from build123d import *

# Parameters (mm, degrees)
F0_W     = 30
F0_H     = 20
F1_DEPTH = 40
F2_R     = 4.672603
F3_DEPTH = 25
F4_R     = 2


with BuildPart() as f1:
    # F0 (on Top) → F1 (new body)
    with BuildSketch(Plane.XY):
        with Locations((15, 10)):
            Rectangle(F0_W, F0_H)
    extrude(amount=F1_DEPTH)

    # F2 (on face) → F3 (join)
    with BuildSketch(Plane.XY.offset(40)):
        with Locations((15, 10)):
            Circle(F2_R)
    extrude(amount=F3_DEPTH)

    # F4
    f4_edges = [f1.edges().sort_by_distance(p)[0] for p in [
        (10.327397, 10, 65),
        (30, 10, 40),
        (15, 0, 40),
        (0, 10, 40),
        (15, 20, 40),
        (30, 20, 20),
        (30, 0, 20),
        (0, 0, 20),
        (0, 20, 20),
    ]]
    fillet(f4_edges, radius=F4_R)


solid = f1.part
Verification items for the finished model (mm, model axes). A direction names the side the tool comes from. Coordinates: 2 decimals unless noted, no trailing zeros. Order: outer loops, then holes, each group sorted by start corner. A loop starts at its lowest first (then second) coordinate and runs counter-clockwise, first axis right, second up.
1. Sectioned sample at D-D, the plane y = 3.5. Record the cut outline in (x, z).
Results found:
outline: (0, 0) - (30, 0) - (30, 38) arc R2 ccw to (28, 40) - (2, 40) arc R2 ccw to (0, 38) - close
2. Set-up check for faces 1 (the face through (15, 0, 19)), 2 (the face through (14.392, 14.633, 51.339)): record each of +Z, -Z, +X, -X, +Y, -Y from which the full face is reachable in a straight line by a thin tool's end or side.
Results found:
face 1: +Z, -Z, +X, -X, -Y
face 2: +Z
3. Scan lines: line 1 (X direction, y = 1.75, z = 23.5); line 2 (Z direction, x = 15.25, y = 16.5); line 3 (X direction, y = 18.75, z = 23.5). Record each from-to range of solid material in increasing order.
Results found:
line 1: x = 0.02 to 29.98
line 2: z = 0 to 40
line 3: x = 0.15 to 29.85
4. Release check for a two-part mould opening along Z. For faces 3 (the face through (15, 10, 0)), 4 (the face through (0, 10, 19)), 5 (the face through (0.57, 10.11, 39.4)) record: +Z half, -Z half, draft (parallel to the pull), parting line (faces both ways), or undercut.
Results found:
face 3: -Z half
face 4: draft
face 5: +Z half
5. Sectioned sample at B-B, the plane x = 15. Record the cut outline in (y, z), and give its area (3 significant figures).
Results found:
outline: (0, 0) - (20, 0) - (20, 38) arc R2 ccw to (18, 40) - (14.67, 40) - (14.67, 63) arc R2 ccw to (12.67, 65) - (7.33, 65) arc R2 ccw to (5.33, 63) - (5.33, 40) - (2, 40) arc R2 ccw to (0, 38) - close
area: 1,030 mm2
6. Go/stop test with flat-tipped pins: pin 1 Ø12 at (x, z) = (21, 56.5) entering from +Y; pin 2 Ø6 at (x, z) = (10, 46) entering from -Y; pin 3 Ø12 at (y, z) = (11, 52) entering from -X. Record where each tip stops, or that it passes through.
Results found:
pin 1: stops at y = 14.67
pin 2: stops at y = 5.78
pin 3: stops at x = 10.33
7. Sectioned sample at C-C, the plane z = 44.5. Record the cut outline in (x, y), and give its area (3 significant figures).
Results found:
outline: circle Ø9.35 at (15, 10)
area: 68.6 mm2
8. Sectioned sample at A-A, the plane y = 10. Record the cut outline in (x, z).
Results found:
outline: (0, 0) - (30, 0) - (30, 38) arc R2 ccw to (28, 40) - (19.67, 40) - (19.67, 63) arc R2 ccw to (17.67, 65) - (12.33, 65) arc R2 ccw to (10.33, 63) - (10.33, 40) - (2, 40) arc R2 ccw to (0, 38) - close
